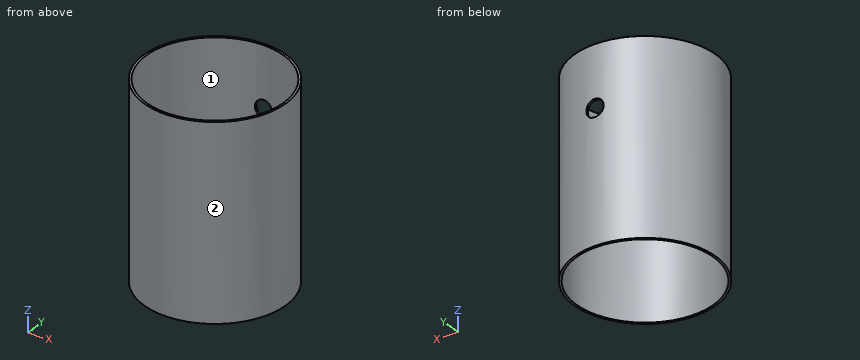
from build123d import *

# Parameters (mm, degrees)
CYLINDER005_R     = 2.75
CYLINDER005_DEPTH = 10
CYLINDER004_R     = 21.5
CYLINDER004_DEPTH = 60
CYLINDER003_R     = 22.2
CYLINDER003_DEPTH = 60


with BuildPart() as cylinder005:
    # Cylinder005 → Cylinder005 (new body)
    with BuildSketch(Plane(origin=(0.5, 26, 66), x_dir=(1, 0, 0), z_dir=(0, -1, 0))):
        Circle(CYLINDER005_R)
    extrude(amount=CYLINDER005_DEPTH)


with BuildPart() as cylinder004:
    # Cylinder004 → Cylinder004 (new body)
    with BuildSketch(Plane.XY):
        Circle(CYLINDER004_R)
    extrude(amount=CYLINDER004_DEPTH)


with BuildPart() as cylindrical_section:
    # Cylinder003 → Cylinder003 (new body)
    with BuildSketch(Plane.XY):
        Circle(CYLINDER003_R)
    extrude(amount=CYLINDER003_DEPTH)

    # Cut002: cut Cylinder004
    add(cylinder004.part, mode=Mode.SUBTRACT)


with BuildPart() as cylindrical_section_1:
    # Cut002 placement: moved
    add(cylindrical_section.part.moved(Location((0, 0, 25))))

    # Cut004: cut Cylinder005
    add(cylinder005.part, mode=Mode.SUBTRACT)


solid = cylindrical_section_1.part
Can you work these out from the model? Positions are in its coordinate system, mm. Face numbers are marked on the shaded views. Give positions to 0.01 mm unless a question says otherwise; leave off trailing zeros. Loops run counter-clockwise (first coordinate to the right, second up) from the corner with the lowest first, then second, coordinate; pieces in that order, holes last. Notation, with made-up numbers: (-17.5, -19) -> (22.5, -19) arc R12 ccw to (22.5, -15) -> close; hole circle Ø2 at (28, 69). An arc over 180 degrees is marked (long way). Use one line per item in the form item = value.
1) If we section it at B-B (x = 2): Please give me the cut outline in (y, z), plus the area to 3 significant figures.
Answers:
outline = (-22.11, 25) -> (-21.41, 25) -> (-21.41, 85) -> (-22.11, 85) -> close; (21.41, 25) -> (22.11, 25) -> (22.11, 63.7) -> (21.41, 63.7) -> close; (21.41, 68.3) -> (22.11, 68.3) -> (22.11, 85) -> (21.41, 85) -> close
area = 81.1 mm²
2) I need wall thicknesses on line 1 along Z through (x, y) = (0.5, 21.8); line 2 along Y through (x, z) = (0, 46.5); line 3 along Y through (x, z) = (11, 65). Which ranges of each line are inside material? Lowest first, please.
Answers:
line_1 = 25 to 63.25, 68.75 to 85
line_2 = -22.2 to -21.5, 21.5 to 22.2
line_3 = -19.28 to -18.47, 18.47 to 19.28
3) If we section it at C-C (z = 76.5): Please give me the cut outline in (x, y).
Answers:
outline = circle Ø44.4 at (0, 0); hole circle Ø43 at (0, 0)
4) If we section it at D-D (y = 5.5): Please give me the cut outline in (x, z).
Answers:
outline = (-21.51, 25) -> (-20.78, 25) -> (-20.78, 85) -> (-21.51, 85) -> close; (20.78, 25) -> (21.51, 25) -> (21.51, 85) -> (20.78, 85) -> close
5) We'd pull the mould along Y, two halves only. Please class the marked faces 1 and 2: released by +Y, released by -Y, zero draft, split by the parting line, or undercut.
Answers:
face_1 = undercut
face_2 = split by the parting line
6) If we section it at A-A (y = 0): Please give me the cut outline in (x, z), plus the area to 3 significant figures.
Answers:
outline = (-22.2, 25) -> (-21.5, 25) -> (-21.5, 85) -> (-22.2, 85) -> close; (21.5, 25) -> (22.2, 25) -> (22.2, 85) -> (21.5, 85) -> close
area = 84.0 mm²
7) Will these pins go through, and if not, where does the flat tip stop? pin 1 (4.5 mm diameter, centred on x = 0.5, z = 66, fed in from -Y); pin 2 (1 mm diameter, centred on x = 7.5, z = 76.5, fed in from +Y); pin 3 (2 mm diameter, centred on x = -3.5, z = 35.5, fed in from +Y).
Answers:
pin_1 = -22.2
pin_2 = 21.07
pin_3 = 22.06
